```python
from build123d import *

# Parameters (mm, degrees)
F0_W     = 41
F0_H     = 52
F1_DEPTH = 3
F3_DEPTH = 3


with BuildPart() as f1:
    # F0 (on Top) → F1 (new body)
    with BuildSketch(Plane.XY):
        with Locations((27.000003, -7.557694)):
            Rectangle(F0_W, F0_H)
    extrude(amount=F1_DEPTH)

    # F2 (on face) → F3 (join)
    with BuildSketch(Plane(origin=(0, 18.442306, 0), x_dir=(-1, 0, 0), z_dir=(0, 1, 0))):
        with BuildLine():
            ThreePointArc((-18.288633, 22.621127), (-17.513213, 24.749818), (-17.250003, 27))
            ThreePointArc((-17.250003, 27), (-27.000003, 36.75), (-36.750003, 27))
            ThreePointArc((-36.750003, 27), (-36.486793, 24.749818), (-35.711373, 22.621127))
            ThreePointArc((-35.711373, 22.621127), (-33.347202, 19.598948), (-30.000003, 17.723012))
            ThreePointArc((-30.000003, 17.723012), (-28.518534, 17.368979), (-27.000003, 17.25))
            ThreePointArc((-27.000003, 17.25), (-25.481473, 17.368979), (-24.000003, 17.723012))
            ThreePointArc((-24.000003, 17.723012), (-20.652805, 19.598948), (-18.288633, 22.621127))
        make_face()
        with BuildLine():
            ThreePointArc((-35.711373, 22.621127), (-36.486793, 24.749818), (-36.750003, 27))
            Line((-36.750003, 27), (-47.500003, 3))
            Line((-47.500003, 3), (-44.500003, 3))
            Line((-44.500003, 3), (-35.711373, 22.621127))
        make_face()
        with BuildLine():
            Line((-24.000003, 3), (-24.000003, 17.723012))
            ThreePointArc((-24.000003, 17.723012), (-25.481473, 17.368979), (-27.000003, 17.25))
            Line((-27.000003, 17.25), (-27.000003, 3))
            Line((-27.000003, 3), (-24.000003, 3))
        make_face()
        with BuildLine():
            ThreePointArc((-27.000003, 17.25), (-28.518534, 17.368979), (-30.000003, 17.723012))
            Line((-30.000003, 17.723012), (-30.000003, 3))
            Line((-30.000003, 3), (-27.000003, 3))
            Line((-27.000003, 3), (-27.000003, 17.25))
        make_face()
        with BuildLine():
            Line((-9.500003, 3), (-6.500003, 3))
            Line((-6.500003, 3), (-17.250003, 27))
            ThreePointArc((-17.250003, 27), (-17.513213, 24.749818), (-18.288633, 22.621127))
            Line((-18.288633, 22.621127), (-9.500003, 3))
        make_face()
    extrude(amount=-F3_DEPTH)


solid = f1.part
```
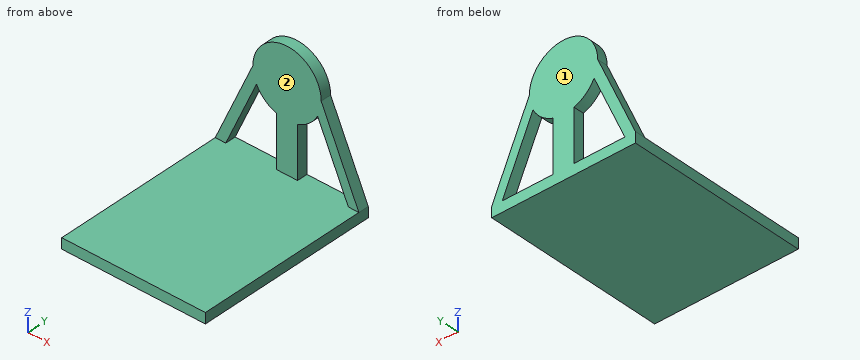
The model under review builds one solid part; all positions refer to its coordinate system, in mm. Face numbers are marked on the shaded views. A direction names the side the tool comes from. Coordinates: 2 decimals unless noted, no trailing zeros. Order: outer loops, then holes, each group sorted by start corner. A loop starts at its lowest first (then second) coordinate and runs counter-clockwise, first axis right, second up. Notation, with made-up numbers: (-7, -32.5) -> (26, -32.5) arc R17 ccw to (26, -25.5) -> close; hole circle Ø2 at (-31.75, -7). An arc over 180 degrees is marked (long way). Answer in a Markdown table with one row per item. Add a question column.
Item 1: Clearance check with flat-ended pins moving along their axes: pin 1 (12.5 mm diameter, centred on x = 20.5, y = 1.5, fed in from +Z); pin 2 (1 mm diameter, centred on x = 19, z = 23.5, fed in from -Y); pin 3 (0.9 mm diameter, centred on y = 17.5, z = 10, fed in from -X). State where each tip first meets the part, or that it passes through.
Item 2: We need section C-C on y = -13. Write out the cut boundary in (x, z).
Item 3: Machinability: for the marked faces 1 and 2, which of the approach directions +Z, -Z, +X, -X, +Y, -Y give a long, thin tool a straight path to every point of the face, cutting with its end or side? Answer none if there is none.
Item 4: We need section B-B on x = 38.5. Write out the cut boundary in (y, z).
Item 5: To check wall thickness, follow probe 1 along X at (y, z) = (16, 15.5); probe 2 along Y at (x, z) = (12.5, 14); probe 3 along Z at (x, y) = (25, -24). State the ranges of each line that lie inside material, in increasing order.
Item 6: We need section D-D on x = 26.5. Write out the cut boundary in (y, z).
Item 7: We need section A-A on z = 6.5. Write out the cut boundary in (x, y), plus the area to 3 significant figures.
Final values:
| question | item | result |
|---|---|---|
| 1 | pin 1 | stops at z = 3 |
| 1 | pin 2 | stops at y = 15.44 |
| 1 | pin 3 | stops at x = 9.43 |
| 2 | outline | (6.5, 0) -> (47.5, 0) -> (47.5, 3) -> (6.5, 3) -> close |
| 3 | face 1 | +Z, -Z, +X, -X, +Y |
| 3 | face 2 | +Z, +X, -X, -Y |
| 4 | outline | (-33.56, 0) -> (18.44, 0) -> (18.44, 3) -> (-33.56, 3) -> close; (15.44, 16.4) -> (18.44, 16.4) -> (18.44, 23.09) -> (15.44, 23.09) -> close |
| 5 | probe 1 | x = 12.1 to 15.1, 24 to 30, 38.9 to 41.9 |
| 5 | probe 2 | y = 15.44 to 18.44 |
| 5 | probe 3 | z = 0 to 3 |
| 6 | outline | (-33.56, 0) -> (18.44, 0) -> (18.44, 36.74) -> (15.44, 36.74) -> (15.44, 3) -> (-33.56, 3) -> close |
| 7 | outline | (8.07, 15.44) -> (11.07, 15.44) -> (11.07, 18.44) -> (8.07, 18.44) -> close; (24, 15.44) -> (30, 15.44) -> (30, 18.44) -> (24, 18.44) -> close; (42.93, 15.44) -> (45.93, 15.44) -> (45.93, 18.44) -> (42.93, 18.44) -> close |
| 7 | area | 36.0 mm2 |
